```python
from build123d import *

# Parameters (mm, degrees)
SCALE1_SCALE = 0.502986482


with BuildPart() as part:
    # Model → Revolve1 (revolve)
    with BuildSketch(Plane.XY):
        with BuildLine():
            Line((28.595574, 124.840746), (28.595574, 131.228004974))
            ThreePointArc((28.595574, 131.228004974), (28.89122421, 131.392844904), (29.188156, 131.555364935))
            Line((29.188156, 131.555364935), (29.188156, 132.16509))
            Line((29.188156, 132.16509), (28.193238, 138.747754))
            Line((28.193238, 138.747754), (23.8331756, 138.747754))
            Line((23.8331756, 138.747754), (22.8382322, 137.752582))
            Line((22.8382322, 137.752582), (22.8382322, 123.845828))
            Line((22.8382322, 123.845828), (23.8331756, 122.850656))
            Line((23.8331756, 122.850656), (25.61082, 122.850656))
            Line((25.61082, 122.850656), (25.61082, 131.570984))
            Line((25.61082, 131.570984), (26.605738, 131.570984))
            Line((26.605738, 131.570984), (26.605738, 123.8885))
            Line((26.605738, 123.8885), (27.813, 123.040902))
            Line((27.813, 123.040902), (27.813, 92.032328))
            Line((27.813, 92.032328), (28.807918, 91.03741))
            Line((28.807918, 91.03741), (32.78632, 91.03741))
            Line((32.78632, 91.03741), (32.78632, 56.684418))
            Line((32.78632, 56.684418), (33.781238, 55.689246))
            Line((33.781238, 55.689246), (38.64991, 55.689246))
            Line((38.64991, 55.689246), (38.64991, 54.101746))
            Line((38.64991, 54.101746), (38.353746, 54.101746))
            Line((38.353746, 54.101746), (37.740082, 53.509418))
            Line((37.740082, 53.509418), (37.740082, 34.416492))
            Line((37.740082, 34.416492), (38.353746, 33.82391))
            Line((38.353746, 33.82391), (39.644828, 33.82391))
            Line((39.644828, 33.82391), (39.644828, 56.684418))
            Line((39.644828, 56.684418), (34.776156, 56.684418))
            Line((34.776156, 56.684418), (34.776156, 94.297754))
            Line((34.776156, 94.297754), (29.993082, 94.297754))
            Line((29.993082, 94.297754), (29.993082, 124.840746))
            Line((29.993082, 124.840746), (28.595574, 124.840746))
        make_face()
    revolve(axis=Axis((49.796303883, 136.783225344, 0), (0, -1, 0)))

    # Model_3 → Revolve2 (revolve)
    with BuildSketch(Plane.XY, mode=Mode.PRIVATE) as revolve2_sk:
        with BuildLine():
            Line((49.796303883, 135.136111003), (49.796303883, 136.783225344))
            ThreePointArc((49.796303883, 136.783225344), (38.838071579, 135.371366431), (28.595574, 131.228004974))
            Line((28.595574, 131.228004974), (49.796303883, 135.136111003))
        make_face()
    revolve(revolve2_sk.sketch.rotate(Axis((49.796303883, 136.783225344, 0), (0, -1, 0)), 180), axis=Axis((49.796303883, 136.783225344, 0), (0, -1, 0)))


with BuildPart() as part_1:
    # Scale1: scaled about (49.796303883, 104.576694566, 0)
    add(part.part.scale(SCALE1_SCALE).moved(Location((24.749436164, 51.976030842, 0))))


solid = part_1.part
```
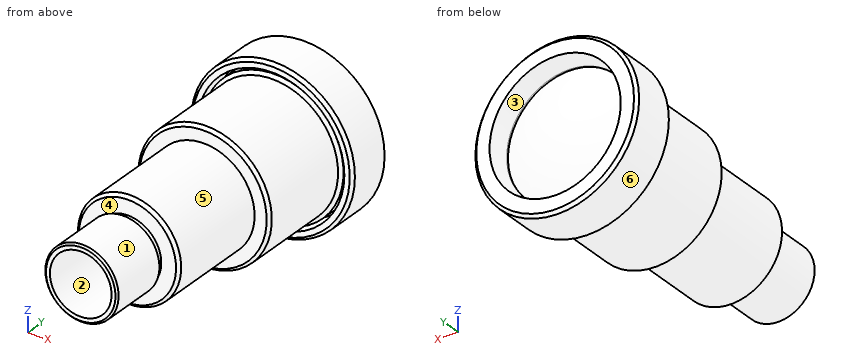
Read the model definition and answer for the solid it produces. Units are mm, in the model's axes. Face numbers are marked on the shaded views. A direction names the side the tool comes from. Give positions to 0.01 mm unless a question says otherwise; leave off trailing zeros. Order: outer loops, then holes, each group sorted by start corner. A loop starts at its lowest first (then second) coordinate and runs counter-clockwise, first axis right, second up.
(1) Find section A-A (y = 116). Give the vertices of the cut face in (x, z), plus the area to 3 significant figures.
(2) For the marked faces 5 and 6, determine the directions among +Z, -Z, +X, -X, +Y, -Y from which every point of the face is accessible in a straight line to the end or side of a thin tool.
(3) Find section C-C (y = 88). Give the vertices of the cut face in (x, z).
(4) For a pull along Z with two mould halves and no side action, classify the marked faces 1, 2, 3 and 4 as released by +Z, released by -Z, zero draft, split by the parting line, or undercut.
(5) Straight lines are drawn through the part: L1, parallel to Z at x = 50, y = 99; L2, parallel to Y at x = 46.25, z = -4.5; L3, parallel to X at y = 87.75, z = 0. For each, find the intervals that lie inside material, in ascending order.
(6) Find section B-B (y = 76.5). Give the vertices of the cut face in (x, z), plus the area to 3 significant figures.
(7) Given pin 1 (6 mm diameter, centred on x = 56.5, y = 112, fed in from -Z); pin 2 (9 mm diameter, centred on x = 52, z = 2.5, fed in from +Y); pin 3 (1 mm diameter, centred on y = 94.5, z = -1.5, fed in from -X), each flat-ended and moving along its own axis, determine where each tip first touches the part or whether it passes through.
Result sheet:
1. outline: circle Ø27.12 at (49.8, 0); circle Ø23.33 at (49.8, 0); hole circle Ø24.33 at (49.8, 0); hole circle Ø21.33 at (49.8, 0)
1. area: 183 mm2
2. face 5: -Y
2. face 6: +Y, -Y
3. outline: circle Ø17.11 at (49.8, 0); hole circle Ø15.11 at (49.8, 0)
4. face 1: split by the parting line
4. face 2: undercut
4. face 3: undercut
4. face 4: zero draft
5. L1: z = -11.06 to -7.55, 7.55 to 11.06
5. L2: y = 68.99 to 79.19, 79.99 to 80.49, 118.89 to 120.01
5. L3: x = 41.24 to 42.24, 57.35 to 58.35
6. outline: circle Ø12.13 at (49.8, 0); hole circle Ø10.21 at (49.8, 0)
6. area: 33.6 mm2
7. pin 1: stops at z = -12.7
7. pin 2: stops at y = 120.78
7. pin 3: stops at x = 41.3
